CAD build for the part. Positions are in the model's coordinates, mm. A direction names the side the tool comes from. Round coordinates to 2 decimals unless told otherwise and drop trailing zeros. Loops run counter-clockwise (first coordinate to the right, second up) from the corner with the lowest first, then second, coordinate; pieces in that order, holes last. Notation, with made-up numbers: (-15.75, -24.5) - (-10.75, -24.5) arc R15 cw to (-10.75, -5.5) - close; hole circle Ø7 at (51, -20.5). An arc over 180 degrees is marked (long way). Use one line per item in the form item = value.
from build123d import *

# Parameters (mm, degrees)
CROQUIS1_R              = 3.5
SALIENTE_EXTRUIR1_DEPTH = 65.5
CORTAR_EXTRUIR3_DEPTH   = 8
CORTAR_EXTRUIR5_START   = -20
CROQUIS7_R              = 3.5
CORTAR_EXTRUIR5_DEPTH   = 20
CROQUIS8_W              = 12.617225576
CROQUIS8_H              = 9.28288649
CORTAR_EXTRUIR6_DEPTH   = 10
SALIENTE_EXTRUIR2_START = 2.5
CROQUIS10_R             = 3.5
SALIENTE_EXTRUIR2_DEPTH = 2.5
CROQUIS11_R             = 3.5
CORTAR_EXTRUIR7_DEPTH   = 1.72


with BuildPart() as part:
    # Croquis1 → Saliente-Extruir1 (new body)
    with BuildSketch(Plane.XY):
        Circle(CROQUIS1_R)
    extrude(amount=-SALIENTE_EXTRUIR1_DEPTH)

    # Croquis6 → Cortar-Extruir3 (cut)
    with BuildSketch(Plane.XY):
        with BuildLine():
            Line((-1.8, 2.045880006), (-1.8, -2.045880006))
            ThreePointArc((-1.8, -2.045880006), (0, -2.725), (1.8, -2.045880006))
            Line((1.8, -2.045880006), (1.8, 2.045880006))
            ThreePointArc((1.8, 2.045880006), (0, 2.725), (-1.8, 2.045880006))
        make_face()
    extrude(amount=-CORTAR_EXTRUIR3_DEPTH, mode=Mode.SUBTRACT)

    # Croquis7 → Cortar-Extruir5 (cut)
    with BuildSketch(Plane(origin=(0, 0, -65.5), x_dir=(-1, 0, 0), z_dir=(0, 0, -1)).offset(CORTAR_EXTRUIR5_START)):
        with Locations(Location((0, 0, 0), (0, 0, 180))):
            Circle(CROQUIS7_R)
        with BuildLine():
            ThreePointArc((1.8, 2.01246118), (0, 2.7), (-1.8, 2.01246118))
            Line((-1.8, 2.01246118), (-1.8, -2.01246118))
            ThreePointArc((-1.8, -2.01246118), (0, -2.7), (1.8, -2.01246118))
            Line((1.8, -2.01246118), (1.8, 2.01246118))
        make_face(mode=Mode.SUBTRACT)
    extrude(amount=CORTAR_EXTRUIR5_DEPTH, mode=Mode.SUBTRACT)

    # Croquis8 → Cortar-Extruir6 (cut)
    with BuildSketch(Plane.ZY.offset(1.8)):
        with Locations((-59.308612788, -0.436721269)):
            Rectangle(CROQUIS8_W, CROQUIS8_H)
    extrude(amount=-CORTAR_EXTRUIR6_DEPTH, mode=Mode.SUBTRACT)

    # Croquis10 → Saliente-Extruir2 (add)
    with BuildSketch(Plane.XY.offset(SALIENTE_EXTRUIR2_START)):
        Circle(CROQUIS10_R)
        with BuildLine():
            Line((-1.8, 2.045880006), (-1.8, -2.045880006))
            ThreePointArc((-1.8, -2.045880006), (0, -2.725), (1.8, -2.045880006))
            Line((1.8, -2.045880006), (1.8, 2.045880006))
            ThreePointArc((1.8, 2.045880006), (0, 2.725), (-1.8, 2.045880006))
        make_face(mode=Mode.SUBTRACT)
    extrude(amount=-SALIENTE_EXTRUIR2_DEPTH)

    # Croquis11 → Cortar-Extruir7 (cut)
    with BuildSketch(Plane.XY.offset(2.5)):
        Circle(CROQUIS11_R)
    extrude(amount=-CORTAR_EXTRUIR7_DEPTH, mode=Mode.SUBTRACT)


solid = part.part
1) Flat gauge pins, fed straight in: pin 1 (1 mm diameter, centred on y = 2.5, z = -17.5, fed in from +X); pin 2 (4 mm diameter, centred on y = -2.5, z = -44, fed in from -X); pin 3 (3 mm diameter, centred on x = -0.5, y = 1, fed in from +Z); pin 4 (2 mm diameter, centred on x = -0.5, y = 0, fed in from +Z). Where does each tip first touch, or does it go through?
Report:
pin_1 = 2.87
pin_2 = -3.46
pin_3 = 0.78
pin_4 = -8
2) Drill centre lines: probe 1 along Y at (x, z) = (-0.25, -2); probe 2 along Z at (x, y) = (-1, 0.5); probe 3 along Z at (x, y) = (-2, -0.5). Where is each one in solid material? Low to high.
Report:
probe_1 = -3.49 to -2.71, 2.71 to 3.49
probe_2 = -53 to -8
probe_3 = -45.5 to 0.78
3) Slice it at A-A (y = 0). Write the cut outline in (x, z), plus the area to 3 significant figures.
Report:
outline = (-3.5, -45.5) - (-1.8, -45.5) - (-1.8, -53) - (1.8, -53) - (1.8, -45.5) - (3.5, -45.5) - (3.5, 0.78) - (1.8, 0.78) - (1.8, -8) - (-1.8, -8) - (-1.8, 0.78) - (-3.5, 0.78) - close
area = 319 mm^2
4) Slice it at B-B (x = 0). Write the cut outline in (y, z) (3 decimals), plus the area to 3 significant figures.
Report:
outline = (-3.5, -45.5) - (-2.7, -45.5) - (-2.7, -53) - (2.7, -53) - (2.7, -45.5) - (3.5, -45.5) - (3.5, 0.78) - (2.725, 0.78) - (2.725, -8) - (-2.725, -8) - (-2.725, 0.78) - (-3.5, 0.78) - close
area = 317 mm^2
5) Tool access for faces 1 (the flat face through (2, 0, -45.5)), 2 (the cylindrical face through (0, -2.7, -49.2)), 3 (the flat face through (0, 0, -8)), 4 (the flat face through (1.8, 0, -49)), 5 (the cylindrical face through (0, 2.7, -49.2)): list every direction of +Z, -Z, +X, -X, +Y, -Y with a clear straight run to the whole face (end or side of a thin tool).
Report:
face_1 = -Z
face_2 = -Z, -Y
face_3 = +Z
face_4 = -Z, +X, +Y, -Y
face_5 = -Z, +Y
6) Two-plate mould, pull along X, no slides. Class faces 6 (the cylindrical face through (3.233, -1.341, -22.036)), 7 (the flat face through (0, 0, -53)), 8 (the cylindrical face through (-0.028, -2.725, -3.549)): +X half, -X half, draft (parallel to the pull), parting line (faces both ways), or undercut.
Report:
face_6 = parting line
face_7 = draft
face_8 = undercut
7) Slice it at C-C (z = -19.5). Write the cut outline in (x, y).
Report:
outline = circle Ø7 at (0, 0)
